Work out the finished part from the listing and answer in its coordinate system (mm). A direction names the side the tool comes from. Round coordinates to 2 decimals unless told otherwise and drop trailing zeros. Loops run counter-clockwise (first coordinate to the right, second up) from the corner with the lowest first, then second, coordinate; pieces in that order, holes last. Notation, with made-up numbers: (16.25, 33.5) -> (39.25, 33.5) arc R4 ccw to (39.25, 39.5) -> close; hole circle Ø8 at (-24, -28.5). An arc over 180 degrees is marked (long way). Use one line per item in the form item = value.
Autodesk Inventor part; units mm, degrees
ref_plane "YZ Plane" through (0, 0, 0) normal (1, 0, 0) x (0, 1, 0)
ref_plane "XZ Plane" through (0, 0, 0) normal (0, 1, 0) x (-1, 0, 0)
ref_plane "XY Plane" through (0, 0, 0) normal (0, 0, 1) x (1, 0, 0)
sketch "Sketch1" plane through (0, 0, 0) normal (1, 0, 0) x (0, 1, 0)
  point P0 (0, 0)
sketch "Sketch2" plane through (0, 0, 0) normal (1, 0, 0) x (0, 1, 0)
  line L0 (0, 0) -> (118, 0)
  line L1 (118, 0) -> (118, -140)
  line L2 (118, -140) -> (0, -140)
  line L3 (0, -140) -> (0, 0)
  circle A0 centre (56, -20) radius 20
  circle A1 centre (56, -20) radius 10
  circle A2 centre (118, -90) radius 15
  circle A3 centre (118, -90) radius 25
  line L4 (118, -115) -> (18, -140)
  line L5 (101, -65) -> (118, -65)
  line L6 (76, -20) -> (76, -40)
  arc A4 (76, -40) -> (101, -65) centre (101, -40) ccw
  point P0 (56, 0)
  dimension "d2" = 40
  dimension "d0" = 140
  dimension "d1" = 118
  dimension "d3" = 20
  dimension "d4" = 30
  dimension "d5" = 50
  dimension "d6" = 56
  dimension "d7" = 56
  dimension "d8" = 20
  dimension "d9" = 20
  dimension "d10" = 50
  dimension "d11" = 50
  dimension "d12" = 18
sketch "Sketch3" plane through (0, 0, 0) normal (0, 0, 1) x (1, 0, 0)
  line L0 (0, 0) -> (-86, 0)
  line L1 (-86, 0) -> (-86, 18)
  line L2 (-86, 18) -> (0, 18)
  line L3 (0, 18) -> (0, 0)
  line L4 (-73, 2) -> (-13, 2)
  line L5 (-43, 18) -> (-43, 0)
  line L6 (-73, 2) -> (-73, 0)
  line L7 (-13, 2) -> (-13, 0)
  point P0 (-43, 2)
  dimension "d14" = 86
  dimension "d15" = 18
  dimension "d16" = 60
  dimension "d17" = 2
extrude "Extrusion1" add sketch "Sketch3" against normal blind 140 contours L0 L7 L4 L5 L2 L3 | L5 L4 L6 L0 L1 L2
extrude "Extrusion2" add sketch "Sketch2" against normal blind 12 contours L0 A0 L6 A4 L5 A3 L4 L2 L3
extrude "Extrusion3" add sketch "Sketch2" against normal blind 30 contours A0
extrude "Extrusion4" add sketch "Sketch2" against normal blind 35 contours A3 L1 A2 | L1 A2 A3
sketch "Sketch4" plane through (-73, 2, 0) normal (0, -1, 0) x (1, 0, 0)
  circle A0 centre (28.7142, -108.9689) radius 5
  circle A1 centre (33.7142, -71.4681) radius 5
  circle A2 centre (21.1452, -46.0088) radius 5
  line L0 (43, 0) -> (43, -40)
  circle A3 centre (43, -35.8595) radius 5
  point P0 (73, 0)
  dimension "d26" = 10
  dimension "d27" = 10
  dimension "d28" = 10
  dimension "d29" = 10
extrude "Extrusion5" cut sketch "Sketch4" against normal blind 18
properties part number "3"
(1) Find section D-D, the plane y = 10. Write down the section's boundary in (x, z).
Completed:
outline = (-86, -140) -> (0, -140) -> (0, 0) -> (-86, 0) -> close; hole circle Ø10 at (-51.85, -46.01); hole circle Ø10 at (-44.29, -108.97); hole circle Ø10 at (-39.29, -71.47); hole circle Ø10 at (-30, -35.86)
(2) For faces 4 (the flat face through (-50, 2, -69)), 5 (the flat face through (-6, 109, -65)), 6 (the flat face through (-35, 129, -101)), determine the directions among +Z, -Z, +X, -X, +Y, -Y from which every point of the face is accessible in a straight line to the end or side of a thin tool.
Completed:
face_4 = +Z, -Z, -Y
face_5 = +Z, +X, -X, +Y
face_6 = +Z, -Z, -X, +Y
(3) Consider L1, parallel to Y at x = -70, z = -31; L2, parallel to X at y = 23.5, z = -18; L3, parallel to Z at x = -24, y = 114.5. Determine where each line is inside the solid, lowest interval first.
Completed:
L1 = 2 to 18
L2 = -12 to 0
L3 = -114.75 to -104.59, -75.41 to -65.25
(4) Given P1, Ø11.5, axis at x = -39.29, z = -71.47, coming from the -Y side; P2, Ø15, axis at y = 121.5, z = -81, coming from the -X side; P3, Ø10, axis at x = -54.5, z = -70.5, coming from the +Y side; P4, Ø18, axis at y = 56, z = -20, coming from the +X side, each flat-ended and moving along its own axis, determine where each tip first touches the part or whether it passes through.
Completed:
P1 = 2
P2 = -35
P3 = 18
P4 = through
(5) Find section A-A, the plane x = -9. Write down the section's boundary in (y, z), then the cut area to 3 significant figures.
Completed:
outline = (0, -140) -> (18, -140) -> (118, -115) arc R25 ccw to (118, -65) -> (101, -65) arc R25 cw to (76, -40) -> (76, -20) arc R20 ccw to (56, 0) -> (0, 0) -> close; hole circle Ø20 at (56, -20); hole circle Ø30 at (118, -90)
area = 12,500 mm2
(6) For a pull along X with two mould halves and no side action, classify faces 1 (the cylindrical face through (-40.37, 9.89, -76.35)), 2 (the flat face through (-79, 0, -69)), 3 (the flat face through (0, 55, -69)) as +X half, -X half, draft (parallel to the pull), parting line (faces both ways), or undercut.
Completed:
face_1 = undercut
face_2 = draft
face_3 = +X half
(7) Find section C-C, the plane y = 125. Write down the section's boundary in (x, z).
Completed:
outline = (-35, -114) -> (0, -114) -> (0, -103.27) -> (-35, -103.27) -> close; (-35, -76.73) -> (0, -76.73) -> (0, -66) -> (-35, -66) -> close
(8) Find section B-B, the plane z = -90. Write down the section's boundary in (x, y).
Completed:
outline = (-86, 0) -> (-73, 0) -> (-73, 2) -> (-13, 2) -> (-13, 0) -> (0, 0) -> (0, 103) -> (-35, 103) -> (-35, 93) -> (-12, 93) -> (-12, 18) -> (-86, 18) -> close; (-35, 133) -> (0, 133) -> (0, 143) -> (-35, 143) -> close
